Part model, mm, in its own coordinate system. Face numbers are marked on the shaded views. A direction names the side the tool comes from. Give positions to 0.01 mm unless a question says otherwise; leave off trailing zeros. Write each loop counter-clockwise with the first axis right and the second up, starting at its lowest first coordinate (ties: lowest second). Pieces come first, ordered by that corner, then holes. Notation, with made-up numbers: (35.5, 16) - (70.5, 16) arc R21 cw to (70.5, 42) - close; hole circle Ø4 at (5, -36). An arc over 180 degrees is marked (long way). Answer as a JSON object with one key per item and string values. Group by question number.
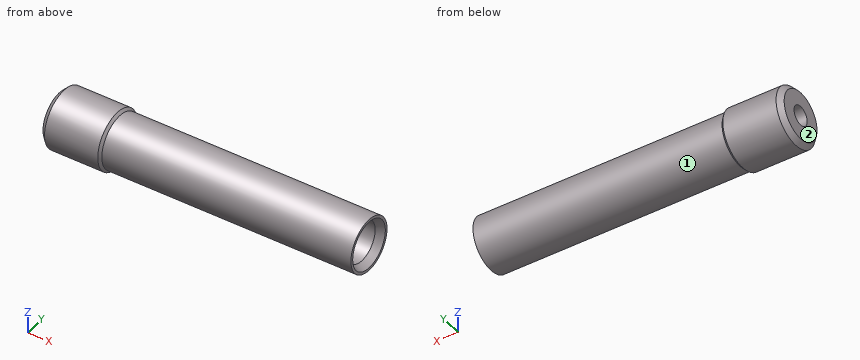
Autodesk Inventor part; units mm, degrees
ref_plane "YZ Plane" through (0, 0, 0) normal (1, 0, 0) x (0, 1, 0)
ref_plane "XZ Plane" through (0, 0, 0) normal (0, 1, 0) x (-1, 0, 0)
ref_plane "XY Plane" through (0, 0, 0) normal (0, 0, 1) x (1, 0, 0)
sketch "Náčrt1" plane through (0, 0, 0) normal (0, 0, 1) x (1, 0, 0)
  line L0 (0, -3.6) -> (0, 0.6)
  line L1 (-6.4, 0) -> (38.4, 0)
  line L2 (0, -1) -> (6, -1)
  line L3 (32, -2.75) -> (6.25, -2.75)
  line L4 (6.25, -2.75) -> (6, -3)
  line L5 (6, -3) -> (0.5, -3)
  line L6 (0.5, -3) -> (0, -2.5)
  line L7 (0, -2.5) -> (0, -1)
  line L8 (32, -2.75) -> (32, -2.05)
  line L9 (6, -1) -> (6.6309, -2.05)
  line L10 (6.6309, -2.05) -> (32, -2.05)
  point P0 (0, 0)
  dimension "d0" = 2
  dimension "d1" = 5.5
  dimension "d3" = 6
  dimension "d4" = 45
  dimension "d5" = 6
  dimension "d6" = 0.5
  dimension "d7" = 90
  dimension "d16" = 4.1
  dimension "d17" = 59
  dimension "d18" = 26
  dimension "d19" = 6
revolve "Rotace1" add sketch "Náčrt1" angle 360 about axis through (-10, 0, 0) along (1, 0, 0)
thread "Závit1"
chamfer "Zkosení1" distance 0.75 angle 30 1 edges at (32, 2.05, 0) measured on face at (15.0873, -2.0235, 0.3288)
1) Drop flat-ended pins along their axis: P1, Ø1.5, axis at x = 26, y = 2.5, coming from the +Z side; P2, Ø2.5, axis at y = 0, z = 0, coming from the +X side; P3, Ø1, axis at x = 27, y = -1, coming from the -Z side. Give the stop position or say it passes through.
2) Saw through at A-A (z = 0). List the corners of the cut face in (x, y), and give its area (4 significant figures).
3) Saw through at C-C (x = 17). List the corners of the cut face in (y, z), and give its area (3 significant figures).
4) Drill centre lines: line 1 along Z through (x, y) = (22, 0); line 2 along Y through (x, z) = (2.85, 0). Where is each one in solid material? Low to high. Write a range as from..to.
5) Saw through at D-D (x = 2.5). List the corners of the cut face in (y, z), and give its area (3 significant figures).
6) Which spindle directions (+Z, -Z, +X, -X, +Y, -Y) get a long thin tool onto all of the face, cutting with end or side? Do the marked faces 1 and 2. Say none if no direction does.
Checks:
{
 "1": {"P1": "z = 2.12", "P2": "x = 6.15", "P3": "z = -2.7"},
 "2": {"outline": "(0, -2.5) - (0.5, -3) - (6, -3) - (6.25, -2.75) - (32, -2.75) - (32, -2.48) - (31.25, -2.05) - (6.63, -2.05) - (6, -1) - (0, -1) - close; (0, 1) - (6, 1) - (6.63, 2.05) - (31.25, 2.05) - (32, 2.48) - (32, 2.75) - (6.25, 2.75) - (6, 3) - (0.5, 3) - (0, 2.5) - close", "area": "60.55 mm2"},
 "3": {"outline": "circle Ø5.5 at (0, 0); hole circle Ø4.1 at (0, 0)", "area": "10.6 mm2"},
 "4": {"line 1": "-2.75..-2.05, 2.05..2.75", "line 2": "-3..-1, 1..3"},
 "5": {"outline": "circle Ø6 at (0, 0); hole circle Ø2 at (0, 0)", "area": "25.1 mm2"},
 "6": {"face 1": "+X", "face 2": "+Z, -Z, -X, +Y, -Y"}
}
